```python
from build123d import *

# Parameters (mm, degrees)
SKETCH1_R           = 100
BOSS_EXTRUDE1_DEPTH = 4
SKETCH2_W           = 4
SKETCH2_H           = 12
SKETCH2_W_2         = 12
SKETCH2_H_2         = 4
CUT_EXTRUDE1_DEPTH  = 4
CUT_EXTRUDE3_START  = -4
SKETCH3_R           = 100
CUT_EXTRUDE3_DEPTH  = 4
SKETCH5_R           = 55
CUT_EXTRUDE4_DEPTH  = 107.986490191
SKETCH6_R           = 1.5
CUT_EXTRUDE5_DEPTH  = 107.986490191
CIRPATTERN1_COUNT   = 8
SKETCH7_R           = 3.5
CUT_EXTRUDE6_DEPTH  = 10
CIRPATTERN2_COUNT   = 4


with BuildPart() as part:
    # Sketch1 → Boss-Extrude1 (new body)
    with BuildSketch(Plane(origin=(0, 0, 0), x_dir=(1, 0, 0), z_dir=(0, 1, 0))):
        with Locations(Location((0, 0, 0), (0, 0, 270))):
            Circle(SKETCH1_R)
    extrude(amount=BOSS_EXTRUDE1_DEPTH)

    # Sketch2 → Cut-Extrude1 (cut)
    with BuildSketch(Plane(origin=(0, 4, 0), x_dir=(1, 0, 0), z_dir=(0, 1, 0))):
        with Locations((-73.597979746, -26)):
            Rectangle(SKETCH2_W, SKETCH2_H)
        with Locations((-73.597979746, 0)):
            Rectangle(SKETCH2_W, SKETCH2_H)
        with Locations((-73.597979746, 26)):
            Rectangle(SKETCH2_W, SKETCH2_H)
        Polygon((-70.426406871, 30.828427125), (-73.254833996, 33.656854249), (-64.769552622, 42.142135624), (-61.941125497, 39.313708499), align=None)
        Polygon((-54.870057685, 46.384776311), (-57.69848481, 49.213203436), (-49.213203436, 57.69848481), (-46.384776311, 54.870057685), align=None)
        Polygon((-39.313708499, 61.941125497), (-42.142135624, 64.769552622), (-33.656854249, 73.254833996), (-30.828427125, 70.426406871), align=None)
        with Locations((-26, 73.597979746)):
            Rectangle(SKETCH2_W_2, SKETCH2_H_2)
        with Locations((0, 73.597979746)):
            Rectangle(SKETCH2_W_2, SKETCH2_H_2)
        with Locations((26, 73.597979746)):
            Rectangle(SKETCH2_W_2, SKETCH2_H_2)
        Polygon((42.142135624, 64.769552622), (39.313708499, 61.941125497), (30.828427125, 70.426406871), (33.656854249, 73.254833996), align=None)
        Polygon((57.69848481, 49.213203436), (54.870057685, 46.384776311), (46.384776311, 54.870057685), (49.213203436, 57.69848481), align=None)
        Polygon((73.254833996, 33.656854249), (70.426406871, 30.828427125), (61.941125497, 39.313708499), (64.769552622, 42.142135624), align=None)
        with Locations((73.597979746, 0)):
            Rectangle(SKETCH2_W, SKETCH2_H)
        with Locations((73.597979746, 26)):
            Rectangle(SKETCH2_W, SKETCH2_H)
        with Locations((73.597979746, -26)):
            Rectangle(SKETCH2_W, SKETCH2_H)
        Polygon((64.769552622, -42.142135624), (61.941125497, -39.313708499), (70.426406871, -30.828427125), (73.254833996, -33.656854249), align=None)
        Polygon((71.597979746, -32), (71.597979746, -29.656854249), (70.426406871, -30.828427125), align=None)
        Polygon((49.213203436, -57.69848481), (46.384776311, -54.870057685), (54.870057685, -46.384776311), (57.69848481, -49.213203436), align=None)
        Polygon((33.656854249, -73.254833996), (30.828427125, -70.426406871), (39.313708499, -61.941125497), (42.142135624, -64.769552622), align=None)
        Polygon((32, -71.597979746), (30.828427125, -70.426406871), (29.656854249, -71.597979746), align=None)
        with Locations((26, -73.597979746)):
            Rectangle(SKETCH2_W_2, SKETCH2_H_2)
        with Locations((0, -73.597979746)):
            Rectangle(SKETCH2_W_2, SKETCH2_H_2)
        with Locations((-26, -73.597979746)):
            Rectangle(SKETCH2_W_2, SKETCH2_H_2)
        Polygon((-29.656854249, -71.597979746), (-30.828427125, -70.426406871), (-32, -71.597979746), align=None)
        Polygon((-30.828427125, -70.426406871), (-33.656854249, -73.254833996), (-42.142135624, -64.769552622), (-39.313708499, -61.941125497), align=None)
        Polygon((-46.384776311, -54.870057685), (-49.213203436, -57.69848481), (-57.69848481, -49.213203436), (-54.870057685, -46.384776311), align=None)
        Polygon((-61.941125497, -39.313708499), (-64.769552622, -42.142135624), (-73.254833996, -33.656854249), (-70.426406871, -30.828427125), align=None)
        Polygon((-70.426406871, -30.828427125), (-71.597979746, -29.656854249), (-71.597979746, -32), align=None)
        Polygon((-71.597979746, 29.656854249), (-70.426406871, 30.828427125), (-71.597979746, 32), align=None)
        Polygon((-29.656854249, 71.597979746), (-32, 71.597979746), (-30.828427125, 70.426406871), align=None)
        Polygon((32, 71.597979746), (29.656854249, 71.597979746), (30.828427125, 70.426406871), align=None)
        Polygon((71.597979746, 32), (70.426406871, 30.828427125), (71.597979746, 29.656854249), align=None)
    extrude(amount=-CUT_EXTRUDE1_DEPTH, mode=Mode.SUBTRACT)

    # Sketch3 → Cut-Extrude3 (cut)
    # profile 1 of 5: a face of its own
    with BuildSketch(Plane(origin=(0, 4, 0), x_dir=(1, 0, 0), z_dir=(0, 1, 0)).offset(CUT_EXTRUDE3_START)):
        Circle(SKETCH3_R)
        Polygon((75.597979746, -32), (32, -75.597979746), (-32, -75.597979746), (-75.597979746, -32), (-75.597979746, 32), (-32, 75.597979746), (32, 75.597979746), (75.597979746, 32), align=None, mode=Mode.SUBTRACT)
    # profile 2 of 5: a face of its own
    with BuildSketch(Plane(origin=(0, 4, 0), x_dir=(1, 0, 0), z_dir=(0, 1, 0)).offset(CUT_EXTRUDE3_START)):
        Polygon((-75.597979746, 32), (-75.597979746, 30.611659087), (-70.199499966, 31.905014714), (-64.769552622, 42.142135624), (-42.142135624, 64.769552622), (-31.064182622, 71.665632478), (-28.788746713, 75.597979746), (-32, 75.597979746), align=None)
    # profile 3 of 5: a face of its own
    with BuildSketch(Plane(origin=(0, 4, 0), x_dir=(1, 0, 0), z_dir=(0, 1, 0)).offset(CUT_EXTRUDE3_START)):
        Polygon((-75.597979746, -32), (-32, -75.597979746), (-29.093903597, -75.597979746), (-30.351010999, -72.169062048), (-42.142135624, -64.769552622), (-64.769552622, -42.142135624), (-71.252442115, -31.167934151), (-75.597979746, -30.54862762), align=None)
    # profile 4 of 5: a face of its own
    with BuildSketch(Plane(origin=(0, 4, 0), x_dir=(1, 0, 0), z_dir=(0, 1, 0)).offset(CUT_EXTRUDE3_START)):
        Polygon((32, -70.176952979), (27.328089277, -75.597979746), (32, -75.597979746), (75.597979746, -32), (75.597979746, -29.546495423), (70.83875298, -31.3565945), (64.769552622, -42.142135624), (42.142135624, -64.769552622), align=None)
    # profile 5 of 5: a face of its own
    with BuildSketch(Plane(origin=(0, 4, 0), x_dir=(1, 0, 0), z_dir=(0, 1, 0)).offset(CUT_EXTRUDE3_START)):
        Polygon((70.83875298, 31.531789385), (75.597979746, 29.562368083), (75.597979746, 32), (32, 75.597979746), (29.807879635, 75.597979746), (31.156089891, 71.258119345), (42.142135624, 64.769552622), (64.769552622, 42.142135624), align=None)
    extrude(amount=CUT_EXTRUDE3_DEPTH, mode=Mode.SUBTRACT)

    # Sketch5 → Cut-Extrude4 (cut, through all)
    with BuildSketch(Plane(origin=(0, 4, 0), x_dir=(1, 0, 0), z_dir=(0, 1, 0))):
        with Locations(Location((0, 0, 0), (0, 0, 270))):
            Circle(SKETCH5_R)
    extrude(amount=-CUT_EXTRUDE4_DEPTH, mode=Mode.SUBTRACT)

    # Sketch6 → Cut-Extrude5 (cut, through all)
    with BuildSketch(Plane(origin=(0, 4, 0), x_dir=(1, 0, 0), z_dir=(0, 1, 0))):
        with Locations(Location((-60.25, 0, 0), (0, 0, 270))):
            Circle(SKETCH6_R)
    cut_extrude5 = extrude(amount=-CUT_EXTRUDE5_DEPTH, mode=Mode.SUBTRACT)

    # CirPattern1: Cut-Extrude5 ×8 about axis
    cirpattern1_axis = Axis((0, 0, 0), (0, 1, 0))
    for i in range(1, CIRPATTERN1_COUNT):
        add(cut_extrude5.rotate(cirpattern1_axis, i * 360 / CIRPATTERN1_COUNT), mode=Mode.SUBTRACT)

    # Sketch7 → Cut-Extrude6 (cut)
    with BuildSketch(Plane(origin=(0, 4, 0), x_dir=(1, 0, 0), z_dir=(0, 1, 0))):
        with BuildLine():
            ThreePointArc((3.5, 60.25), (0, 56.75), (-3.5, 60.25))
            Line((-3.5, 60.25), (-3.5, 54.888523391))
            ThreePointArc((-3.5, 54.888523391), (0, 55), (3.5, 54.888523391))
            Line((3.5, 54.888523391), (3.5, 60.25))
        make_face()
        with Locations((0, 60.25)):
            Circle(SKETCH7_R)
    cut_extrude6 = extrude(amount=-CUT_EXTRUDE6_DEPTH, mode=Mode.SUBTRACT)

    # CirPattern2: Cut-Extrude6 ×4 about axis
    cirpattern2_axis = Axis((0, 0, 0), (0, 1, 0))
    for i in range(1, CIRPATTERN2_COUNT):
        add(cut_extrude6.rotate(cirpattern2_axis, i * 360 / CIRPATTERN2_COUNT), mode=Mode.SUBTRACT)


solid = part.part
```
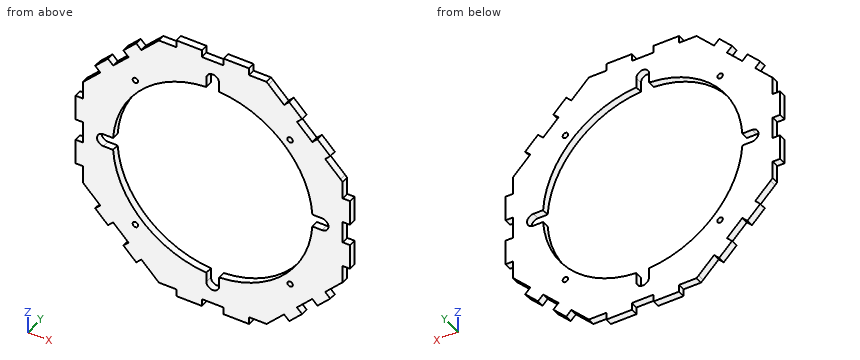
The listing builds one solid part. Answer for the finished solid, in the listing's coordinates (mm). Round coordinates to 2 decimals unless told otherwise and drop trailing zeros. Loops run counter-clockwise (first coordinate to the right, second up) from the corner with the lowest first, then second, coordinate; pieces in that order, holes last.
Q1. Given pin 1 Ø1.2 at (x, y) = (-73, 1.5) entering from +Z; pin 2 Ø1.2 at (y, z) = (2.5, 1) entering from -X; pin 3 Ø1.2 at (y, z) = (1, 74) entering from +X, each flat-ended and moving along its own axis, determine where each tip first touches the part or whether it passes through.
Q2. Section C-C, the plane y = 3.1 is taken. Count the separate pieces of the cut face and the enclosed holes in it, then the cut area to 3 significant figures.
Q3. Section A-A, the plane z = 0 is taken. Determine the outline of the cut face in (x, y).
Q4. Section B-B, the plane x = 15.5 is taken. Determine the outline of the cut face in (y, z).
Q5. Find the intervals of material crossed by line 1 (Z direction, x = -47, y = 3.6); line 2 (Z direction, x = -4, y = 2.25); line 3 (Z direction, x = 0, y = 3.35), in increasing order.
Completed:
1. pin 1: stops at z = 20
1. pin 2: stops at x = -71.6
1. pin 3: stops at x = 20
2. separate pieces: 1
2. enclosed holes: 5
2. area: 8,000 mm2
3. outline: (-71.6, 0) - (-63.75, 0) - (-63.75, 4) - (-71.6, 4) - close; (63.75, 0) - (71.6, 0) - (71.6, 4) - (63.75, 4) - close
4. outline: (0, -75.6) - (4, -75.6) - (4, -52.77) - (0, -52.77) - close; (0, 52.77) - (4, 52.77) - (4, 75.6) - (0, 75.6) - close
5. line 1: z = -59.91 to -55.49, -54.25 to -28.57, 28.57 to 54.25, 55.49 to 59.91
5. line 2: z = -71.6 to -54.85, 54.85 to 71.6
5. line 3: z = -71.6 to -63.75, 63.75 to 71.6
